Input: part model. Units: mm. Frame: model coordinates. Face numbers are marked on the shaded views. A direction names the side the tool comes from. Coordinates: 2 decimals unless noted, no trailing zeros. Order: outer loops, then holes, each group sorted by start corner. A loop starts at its lowest first (then second) coordinate and runs counter-clockwise, first axis right, second up. Notation, with made-up numbers: (-11.75, 47.25) -> (34.25, 47.25) arc R19 cw to (34.25, 73.25) -> close; hole circle Ø8 at (37, -21.75). An arc over 180 degrees is marked (long way). Write each question's results on one line, items separated by ' | '.
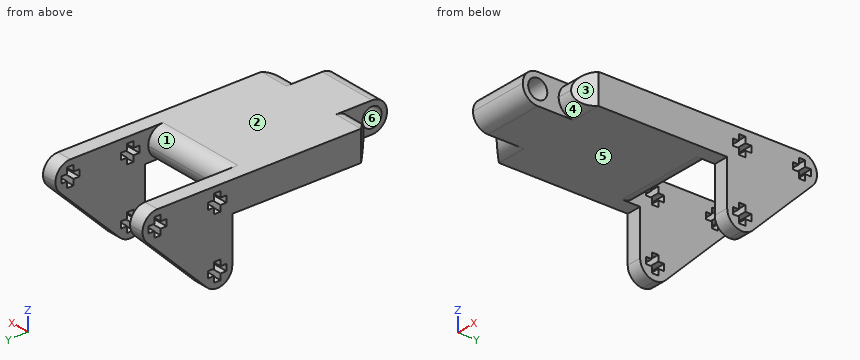
```python
from build123d import *

# Parameters (mm, degrees)
F1_DEPTH = 7.9375
F2_R     = 3.96874
F3_W     = 3.96875
F3_H     = 23.8125
F4_DEPTH = 15.875
F5_W     = 1.56845
F5_H     = 1.6891
F5_W_2   = 1.6891
F5_H_2   = 1.56845
F5_R     = 2.54
F6_DEPTH = 31.75
F8_DEPTH = 7.9375


# Not quite as in the source:
# - a fillet or chamfer is up to 0.001 mm smaller than in the source, because OpenCascade refuses the exact size


with BuildPart() as f1:
    # F0 (on Top) → F1 (new body)
    with BuildSketch(Plane.XY):
        Polygon((0, 0), (0, -9.525), (15.875, -9.525), (15.875, 0), (23.8125, 0), (23.8125, 61.9125), (19.84375, 61.9125), (19.84375, 37.30625), (-3.96875, 37.30625), (-3.96875, 61.9125), (-7.9375, 61.9125), (-7.9375, 0), align=None)
    extrude(amount=F1_DEPTH)

    # F2 (radius 3.96875 in the source; OpenCascade refuses exactly that, so slightly less here)
    f2_edges = [f1.edges().sort_by_distance(p)[0] for p in [
        (19.84375, 0, 7.9375),
        (19.84375, 0, 0),
        (7.9375, -9.525, 0),
        (7.9375, -9.525, 7.9375),
        (-3.96875, 0, 7.9375),
        (-3.96875, 0, 0),
        (-5.953125, 61.9125, 7.9375),
        (7.9375, 37.30625, 0),
        (7.9375, 37.30625, 7.9375),
        (21.828125, 61.9125, 7.9375),
    ]]
    fillet(f2_edges, radius=F2_R)

    # F3 (on face) → F4 (join)
    with BuildSketch(Plane(origin=(0, 0, 0), x_dir=(1, 0, 0), z_dir=(0, 0, -1))):
        with Locations((21.828125, -50.00625)):
            Rectangle(F3_W, F3_H)
        with Locations((-5.953125, -50.00625)):
            Rectangle(F3_W, F3_H)
    extrude(amount=F4_DEPTH)

    # F5 (on face) → F6 (cut, through all)
    with BuildSketch(Plane.YZ.offset(23.8125)):
        with BuildLine():
            Line((38.1, -15.875), (42.06875, -15.875))
            ThreePointArc((42.06875, -15.875), (39.2624199622, -14.7125800378), (38.1, -11.90625))
            Line((38.1, -11.90625), (38.1, -15.875))
        make_face()
        with BuildLine():
            Line((42.06875, -15.875), (61.9125, -15.875))
            Line((61.9125, -15.875), (61.9125, 3.96875))
            ThreePointArc((61.9125, 3.96875), (61.6103968947, 2.4499751278), (60.7500800378, 1.1624199622))
            Line((60.7500800378, 1.1624199622), (44.8750800378, -14.7125800378))
            ThreePointArc((44.8750800378, -14.7125800378), (43.5875248722, -15.5728968947), (42.06875, -15.875))
        make_face()
        with Locations((43.697525, -11.90625)):
            Rectangle(F5_W, F5_H)
        with Locations((42.06875, -11.90625)):
            Rectangle(F5_W_2, F5_H)
        with Locations((42.06875, -10.277475)):
            Rectangle(F5_W_2, F5_H_2)
        with Locations((40.439975, -11.90625)):
            Rectangle(F5_W, F5_H)
        with Locations((42.06875, -13.535025)):
            Rectangle(F5_W_2, F5_H_2)
        with Locations((57.94375, 5.597525)):
            Rectangle(F5_W_2, F5_H_2)
        with Locations((57.94375, 3.96875)):
            Rectangle(F5_W_2, F5_H)
        with Locations((56.314975, 3.96875)):
            Rectangle(F5_W, F5_H)
        with Locations((59.572525, 3.96875)):
            Rectangle(F5_W, F5_H)
        with Locations((57.94375, 2.339975)):
            Rectangle(F5_W_2, F5_H_2)
        with Locations((42.06875, 2.339975)):
            Rectangle(F5_W_2, F5_H_2)
        with Locations((42.06875, 3.96875)):
            Rectangle(F5_W_2, F5_H)
        with Locations((43.697525, 3.96875)):
            Rectangle(F5_W, F5_H)
        with Locations((40.439975, 3.96875)):
            Rectangle(F5_W, F5_H)
        with Locations((42.06875, 5.597525)):
            Rectangle(F5_W_2, F5_H_2)
        with Locations((-5.55625, 3.96875)):
            Circle(F5_R)
    extrude(amount=-F6_DEPTH, mode=Mode.SUBTRACT)

    # F7 (on face) → F8 (cut, through all)
    with BuildSketch(Plane.XY.offset(7.9375)):
        Polygon((19.84375, 0), (23.8125, 0), (23.8125, 3.96875), align=None)
        Polygon((-7.9375, 3.96875), (-7.9375, 0), (-3.96875, 0), align=None)
    extrude(amount=-F8_DEPTH, mode=Mode.SUBTRACT)


solid = f1.part
```
(1) Cut plane C-C, the plane z = -10.25. Return loops of the section in (x, y), plus the area to 3 significant figures.
Return value:
outline: (-7.94, 38.1) -> (-3.97, 38.1) -> (-3.97, 41.22) -> (-7.94, 41.22) -> close; (-7.94, 42.91) -> (-3.97, 42.91) -> (-3.97, 49.34) -> (-7.94, 49.34) -> close; (19.84, 38.1) -> (23.81, 38.1) -> (23.81, 41.22) -> (19.84, 41.22) -> close; (19.84, 42.91) -> (23.81, 42.91) -> (23.81, 49.34) -> (19.84, 49.34) -> close | area: 75.8 mm2
(2) Pin query (flat end, axial travel): P1, Ø10, axis at x = 0.5, y = 53, coming from the -Z side; P2, Ø8.5, axis at y = -3, z = 2.5, coming from the +X side; P3, Ø3, axis at x = 16.5, z = 5, coming from the -Y side (3 decimals); P4, Ø0.5, axis at x = -5.5, y = 56, coming from the -Z side. Return the tip coordinate at first contact, or that it passes through.
Return value:
P1: z = -8.83 | P2: x = 21.09 | P3: y = -9.525 | P4: z = -3.84
(3) Cut plane D-D, the plane y = -4. Return loops of the section in (x, z) (1 decimal), plus the area to 3 significant figures.
Return value:
outline: (0, 0) -> (15.9, 0) -> (15.9, 2) -> (0, 2) -> close; (0, 6) -> (15.9, 6) -> (15.9, 7.9) -> (0, 7.9) -> close | area: 62.3 mm2
(4) Line query: line 1 along Z through (x, y) = (-6, 44); line 2 along Z through (x, y) = (7.5, 11); line 3 along X through (y, z) = (45, 4). Output: solid intervals per line, ascending. Write a range as from..to.
Return value:
line 1: -15.37..-12.75, -11.06..3.12, 4.81..7.94 | line 2: 0..7.94 | line 3: -7.94..-3.97, 19.84..23.81
(5) Reachability of the marked faces 4, 5 and 6 from +Z, -Z, +X, -X, +Y, -Y: full face, straight path, thin tool, end or side. Return the list, or none.
Return value:
face 4: -Z, +X, -Y | face 5: -Z, +X, -X, -Y | face 6: +X, -X
(6) Mould query, pull axis X, two halves, no side actions, for the marked faces 1, 2 and 3. Classes: +X half, -X half, draft (parallel to the pull), parting line (faces both ways), or undercut.
Return value:
face 1: undercut | face 2: draft | face 3: +X half
(7) Cut plane B-B, the plane z = -1. Return loops of the section in (x, y), plus the area to 3 significant figures.
Return value:
outline: (-7.94, 38.1) -> (-3.97, 38.1) -> (-3.97, 58.59) -> (-7.94, 58.59) -> close; (19.84, 38.1) -> (23.81, 38.1) -> (23.81, 58.59) -> (19.84, 58.59) -> close | area: 163 mm2
